```python
from build123d import *

# Parameters (mm, degrees)
F0_R     = 1.75
F1_DEPTH = 2


with BuildPart() as f1:
    # F0 (on Top) → F1 (new body)
    with BuildSketch(Plane.XY):
        with BuildLine():
            Line((57.7837471709, 69.5580622628), (-34.7162528291, 69.5580622628))
            Line((-34.7162528291, 69.5580622628), (-34.7162528291, 42.5580622628))
            Line((-34.7162528291, 42.5580622628), (-43.2162528291, 42.5580622628))
            Line((-43.2162528291, 42.5580622628), (-43.2162528291, 5.0580622628))
            Line((-43.2162528291, 5.0580622628), (-34.7162528291, 5.0580622628))
            Line((-34.7162528291, 5.0580622628), (-34.7162528291, -22.9419377372))
            Line((-34.7162528291, -22.9419377372), (57.7837471709, -22.9419377372))
            Line((57.7837471709, -22.9419377372), (57.7837471709, 5.0580622628))
            Line((57.7837471709, 5.0580622628), (61.776727438, 5.0580622628))
            Line((61.776727438, 5.0580622628), (61.7764500569, 6.9623562581))
            ThreePointArc((61.7764500569, 6.9623562581), (60.5385780505, 9.9496128474), (63.5261951319, 8.712611146))
            Line((63.5261951319, 8.712611146), (66.3054800854, 8.713015979))
            Line((66.3054800854, 8.713015979), (66.3054800854, 42.5580622628))
            Line((66.3054800854, 42.5580622628), (57.7837471709, 42.5580622628))
            Line((57.7837471709, 42.5580622628), (57.7837471709, 69.5580622628))
        make_face()
        with Locations((-36.9397651508, 8.7772880495)):
            Circle(F0_R, mode=Mode.SUBTRACT)
        with Locations((-36.9361157864, 38.7772880495)):
            Circle(F0_R, mode=Mode.SUBTRACT)
        with Locations((61.7687867672, 38.9017461427)):
            Circle(F0_R, mode=Mode.SUBTRACT)
        with BuildLine():
            Line((66.3054800854, 5.0580622628), (66.3054800854, 8.713015979))
            Line((66.3054800854, 8.713015979), (63.5261951319, 8.712611146))
            ThreePointArc((63.5261951319, 8.712611146), (63.5261951458, 8.7124836928), (63.5261951505, 8.7123562396))
            ThreePointArc((63.5261951505, 8.7123562396), (63.0137221373, 7.4750094988), (61.7764500569, 6.9623562581))
            Line((61.7764500569, 6.9623562581), (61.776727438, 5.0580622628))
            Line((61.776727438, 5.0580622628), (66.3054800854, 5.0580622628))
        make_face()
    extrude(amount=F1_DEPTH)


solid = f1.part
```
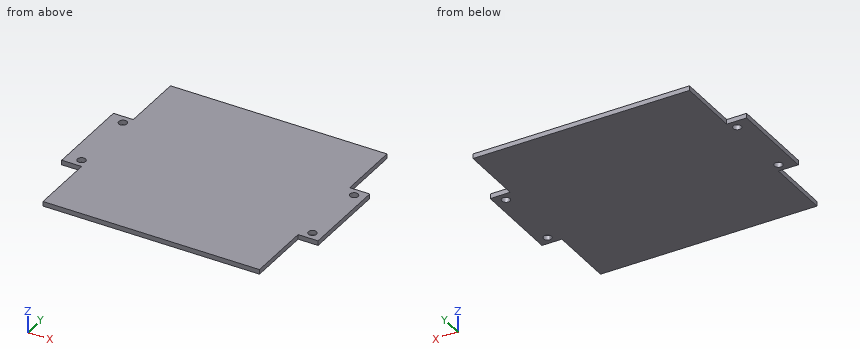
Model file for the job. Use its own axes, mm. Coordinates: 2 decimals unless noted, no trailing zeros. Write each loop counter-clockwise with the first axis right and the second up, starting at its lowest first coordinate (ties: lowest second). Pieces come first, ordered by that corner, then holes. Notation, with made-up numbers: (85, 48) - (115, 48) arc R19 cw to (115, 67) - close; hole circle Ø10 at (-9.5, 40). An arc over 180 degrees is marked (long way). Use a Markdown table: item, result. Add a question column.
Item 1: Drill centre lines: line 1 along Y through (x, z) = (60.5, 0.8); line 2 along X through (y, z) = (38.5, 1.6); line 3 along X through (y, z) = (-13.5, 0.45). Where is each one in solid material? Low to high.
Item 2: Band-saw the part on A-A, the plane z = 0.4. Give the number of separate pieces and of enclosed holes in the cut face, and give its area (3 significant figures).
Item 3: Drop flat-ended pins along their axis: pin 1 (1 mm diameter, centred on y = 55.5, z = 1.5, fed in from -X); pin 2 (2 mm diameter, centred on x = 61.77, y = 38.9, fed in from -Z); pin 3 (0.6 mm diameter, centred on y = 49.5, z = 1.5, fed in from +X); pin 4 (1 mm diameter, centred on x = 64, z = 1, fed in from +Y). Give the stop position or say it passes through.
Item 4: Band-saw the part on B-B, the plane y = -12. Write the cut outline in (x, z).
A:
| question | item | result |
|---|---|---|
| 1 | line 1 | y = 5.06 to 7.51, 9.91 to 37.7, 40.11 to 42.56 |
| 1 | line 2 | x = -43.22 to -38.66, -35.21 to 60.07, 63.47 to 66.31 |
| 1 | line 3 | x = -34.72 to 57.78 |
| 2 | separate pieces | 1 |
| 2 | enclosed holes | 4 |
| 2 | area | 9,160 mm² |
| 3 | pin 1 | stops at x = -34.72 |
| 3 | pin 2 | passes through |
| 3 | pin 3 | stops at x = 57.78 |
| 3 | pin 4 | stops at y = 42.56 |
| 4 | outline | (-34.72, 0) - (57.78, 0) - (57.78, 2) - (-34.72, 2) - close |
